Part model, mm, in its own coordinate system. Face numbers are marked on the shaded views. A direction names the side the tool comes from. Coordinates: 2 decimals unless noted, no trailing zeros. Order: outer loops, then holes, each group sorted by start corner. A loop starts at its lowest first (then second) coordinate and runs counter-clockwise, first axis right, second up. Notation, with made-up numbers: M 55.5,19.25 L 70.5,19.25 A30 cw 70.5,56.25 Z; hole C 16,-21 d2. An arc over 180 degrees is marked long. Answer in a Markdown table with one row per item. Add a question column.
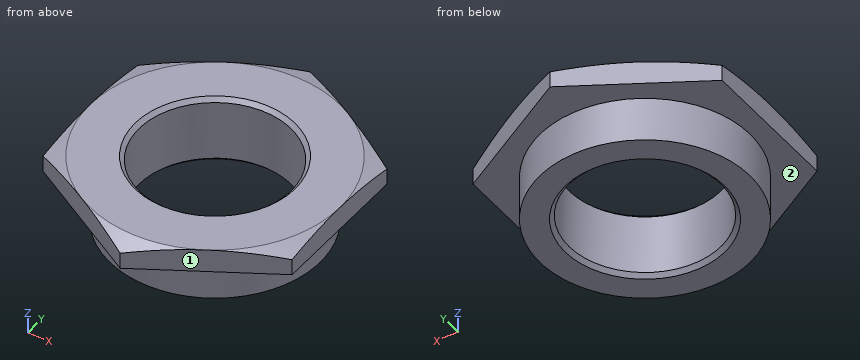
from build123d import *

# Parameters (mm, degrees)
EXTRUDE1_DEPTH      = 2.159
SKETCH14_OUTSIDE_W  = 12.402
SKETCH14_OUTSIDE_H  = 13.63
SKETCH14_OUTSIDE_R  = 3.3401
CUT_EXTRUDE7_DEPTH  = 1.4224
SKETCH7_R           = 2.413
CUT_EXTRUDE3_DEPTH  = 7.435336794
SKETCH20_OUTSIDE_W  = 53.258
SKETCH20_OUTSIDE_H  = 54.486
SKETCH20_OUTSIDE_R  = 3.96875
CUT_EXTRUDE13_DEPTH = 7.435336794
CUT_EXTRUDE13_DRAFT = -70


with BuildPart() as part:
    # Sketch1 → Extrude1 (new body)
    with BuildSketch(Plane.XY):
        Polygon((0, 4.582717762), (-3.96875, 2.291358881), (-3.96875, -2.291358881), (0, -4.582717762), (3.96875, -2.291358881), (3.96875, 2.291358881), align=None)
    extrude(amount=-EXTRUDE1_DEPTH)

    # Sketch14 outside → Cut-Extrude7 (cut)
    with BuildSketch(Plane(origin=(0, 0, -2.159), x_dir=(-1, 0, 0), z_dir=(0, 0, -1))):
        Rectangle(SKETCH14_OUTSIDE_W, SKETCH14_OUTSIDE_H)
        Circle(SKETCH14_OUTSIDE_R, mode=Mode.SUBTRACT)
    extrude(amount=-CUT_EXTRUDE7_DEPTH, mode=Mode.SUBTRACT)

    # Sketch7 → Cut-Extrude3 (cut, through all)
    with BuildSketch(Plane.XY):
        Circle(SKETCH7_R)
    extrude(amount=-CUT_EXTRUDE3_DEPTH, mode=Mode.SUBTRACT)

    # Cut-Extrude6 cone 1 section (through the dimple's axis) → Cut-Extrude6 (revolve, cut)
    with BuildSketch(Plane(origin=(0, 0, 0), x_dir=(0, -1, 0), z_dir=(1, 0, 0))):
        Polygon((0, 0), (2.54, 0), (0, 2.54), align=None)
    revolve(axis=Axis((0, 0, 0), (0, 0, -1)), mode=Mode.SUBTRACT)

    # Cut-Extrude11 cone 1 section (through the dimple's axis) → Cut-Extrude11 (revolve, cut)
    with BuildSketch(Plane(origin=(0, 0, -2.159), x_dir=(0, 1, 0), z_dir=(1, 0, 0))):
        Polygon((0, 0), (2.54, 0), (0, 2.54), align=None)
    revolve(axis=Axis((0, 0, -2.159), (0, 0, 1)), mode=Mode.SUBTRACT)


with BuildPart() as cut_extrude13_tool:
    # Sketch20 outside → Cut-Extrude13 (with draft: the straight prism first)
    with BuildSketch(Plane.XY):
        Rectangle(SKETCH20_OUTSIDE_W, SKETCH20_OUTSIDE_H)
        Circle(SKETCH20_OUTSIDE_R, mode=Mode.SUBTRACT)
    extrude(amount=-CUT_EXTRUDE13_DEPTH)
    # Cut-Extrude13: the draft: its side faces are tilted about the plane it starts from
    cut_extrude13_sides = [cut_extrude13_tool.faces().sort_by_distance(p)[0] for p in [
        (0, -27.243, -3.717668397),
        (26.629, 0, -3.717668397),
        (0, 27.243, -3.717668397),
        (-26.629, 0, -3.717668397),
        (-3.96875, 0, -3.717668397),
    ]]
    draft(cut_extrude13_sides, Plane.XY, CUT_EXTRUDE13_DRAFT)


with BuildPart() as part_1:
    add(part.part)

    # Cut-Extrude13: cut by cut_extrude13_tool
    add(cut_extrude13_tool.part, mode=Mode.SUBTRACT)


solid = part_1.part
(1) Slice it at A-A (z = -0.4). List the corners of the cut face in (x, y).
(2) Slice it at B-B (z = -1.75). List the corners of the cut face in (x, y).
(3) Wall check: line 1 (Y direction, x = 0, z = -0.8); line 2 (X direction, y = 0, z = -0.7); line 3 (X direction, y = 0.75, z = -0.6). Give the ranges that are in metal, low to high.
(4) 3-axis set-ups, long thin cutter, end or side, ignore diameter. For the marked faces 1 and 2: which of +Z, -Z, +X, -X, +Y, -Y reach the whole face in a straight line?
Computed:
| question | item | result |
|---|---|---|
| 1 | outline | M -3.97,-2.29 L 0,-4.58 L 3.97,-2.29 L 3.97,2.29 L 0,4.58 L -3.97,2.29 Z; hole C 0,0 d4.83 |
| 2 | outline | C 0,0 d6.68; hole C 0,0 d4.83 |
| 3 | line 1 | y = -3.34 to -2.41, 2.41 to 3.34 |
| 3 | line 2 | x = -3.97 to -2.41, 2.41 to 3.97 |
| 3 | line 3 | x = -3.97 to -2.29, 2.29 to 3.97 |
| 4 | face 1 | +Z, -Z, +X, -Y |
| 4 | face 2 | -Z |
